Can you work these out from the model? Positions are in its coordinate system, mm. Coordinates: 2 decimals unless noted, no trailing zeros. Order: outer loops, then holes, each group sorted by start corner. A loop starts at its lowest first (then second) coordinate and runs counter-clockwise, first axis right, second up. Notation, with made-up numbers: (54.5, 60) -> (66.5, 60) arc R22 ccw to (66.5, 69) -> close; hole circle Ø2 at (26, 34). An arc over 180 degrees is marked (long way). Write item = value, one per line.
```python
from build123d import *

# Parameters (mm, degrees)
F0_W     = 60
F0_H     = 110
F1_DEPTH = 5
F2_D     = 8.5
F3_D     = 10.5
F4_D     = 3.5
F5_R     = 10
F6_R     = 20


with BuildPart() as f1:
    # F0 (on Top) → F1 (new body)
    with BuildSketch(Plane.XY):
        with Locations((0, 30)):
            Rectangle(F0_W, F0_H)
    extrude(amount=F1_DEPTH)

    # F2 (through all)
    with Locations(Plane(origin=(0, 0, 0), x_dir=(1, 0, 0), z_dir=(0, 0, -1))):
        with Locations((-20, 15), (20, 15)):
            Hole(F2_D / 2)

    # F3 (through all)
    with Locations(Plane(origin=(0, 0, 0), x_dir=(1, 0, 0), z_dir=(0, 0, -1))):
        with Locations((-12, -45)):
            Hole(F3_D / 2)

    # F4 (through all)
    with Locations(Plane(origin=(0, 0, 0), x_dir=(1, 0, 0), z_dir=(0, 0, -1))):
        with Locations((5, -65), (22, -35)):
            Hole(F4_D / 2)

    # F5
    f5_edges = [f1.edges().sort_by_distance(p)[0] for p in [
        (-30, -25, 2.5),
        (30, -25, 2.5),
    ]]
    fillet(f5_edges, radius=F5_R)

    # F6
    f6_edges = [f1.edges().sort_by_distance(p)[0] for p in [
        (-30, 85, 2.5),
        (30, 85, 2.5),
    ]]
    fillet(f6_edges, radius=F6_R)


solid = f1.part
```
Item 1: I want a section at D-D, the plane x = 22. Please give me the cut outline in (y, z).
A:
outline = (-24.8, 0) -> (-18.75, 0) -> (-18.75, 5) -> (-24.8, 5) -> close; (-11.25, 0) -> (33.25, 0) -> (33.25, 5) -> (-11.25, 5) -> close; (36.75, 0) -> (81, 0) -> (81, 5) -> (36.75, 5) -> close
Item 2: If I drill on probe 1 along X at (y, z) = (35, 2.55); probe 2 along Y at (x, z) = (5, 2.3); probe 3 along X at (y, z) = (-12, 2.9), over which ranges is the centre line in solid material (lowest first)?
A:
probe_1 = -30 to 20.25, 23.75 to 30
probe_2 = -25 to 63.25, 66.75 to 85
probe_3 = -30 to -23.01, -16.99 to 16.99, 23.01 to 30
Item 3: I want a section at C-C, the plane z = 1.45. Please give me the cut outline in (x, y), plus the area to 3 significant figures.
A:
outline = (-30, -15) arc R10 ccw to (-20, -25) -> (20, -25) arc R10 ccw to (30, -15) -> (30, 65) arc R20 ccw to (10, 85) -> (-10, 85) arc R20 ccw to (-30, 65) -> close; hole circle Ø8.5 at (-20, -15); hole circle Ø10.5 at (-12, 45); hole circle Ø3.5 at (5, 65); hole circle Ø8.5 at (20, -15); hole circle Ø3.5 at (22, 35)
area = 6,170 mm2
Item 4: I want a section at A-A, the plane y = 45. Please give me the cut outline in (x, z), plus the area to 4 significant figures.
A:
outline = (-30, 0) -> (-17.25, 0) -> (-17.25, 5) -> (-30, 5) -> close; (-6.75, 0) -> (30, 0) -> (30, 5) -> (-6.75, 5) -> close
area = 247.5 mm2
Item 5: If we mould it in two halves opening along X, with no side actions, what happens to faces 1 (the cylindrical face through (20.92, -10.85, 2.53)), 2 (the flat face through (-30, 24, 2)), 3 (the flat face through (0, 31, 0))? For each: pulls with the +X half, pulls with the -X half, needs draft (parallel to the pull), parting line crosses it, or undercut.
A:
face_1 = undercut
face_2 = pulls with the -X half
face_3 = needs draft
Item 6: I want a section at B-B, the plane x = 5. Please give me the cut outline in (y, z).
A:
outline = (-25, 0) -> (63.25, 0) -> (63.25, 5) -> (-25, 5) -> close; (66.75, 0) -> (85, 0) -> (85, 5) -> (66.75, 5) -> close
